Study the drawing (mm; zero at the part's minimum x, y, z) and answer. Coordinates: 2 decimals unless noted, no trailing zeros. Order: outer loops, then holes, each group sorted by start corner. A loop starts at its lowest first (then second) coordinate and runs counter-clockwise, first axis right, second up.
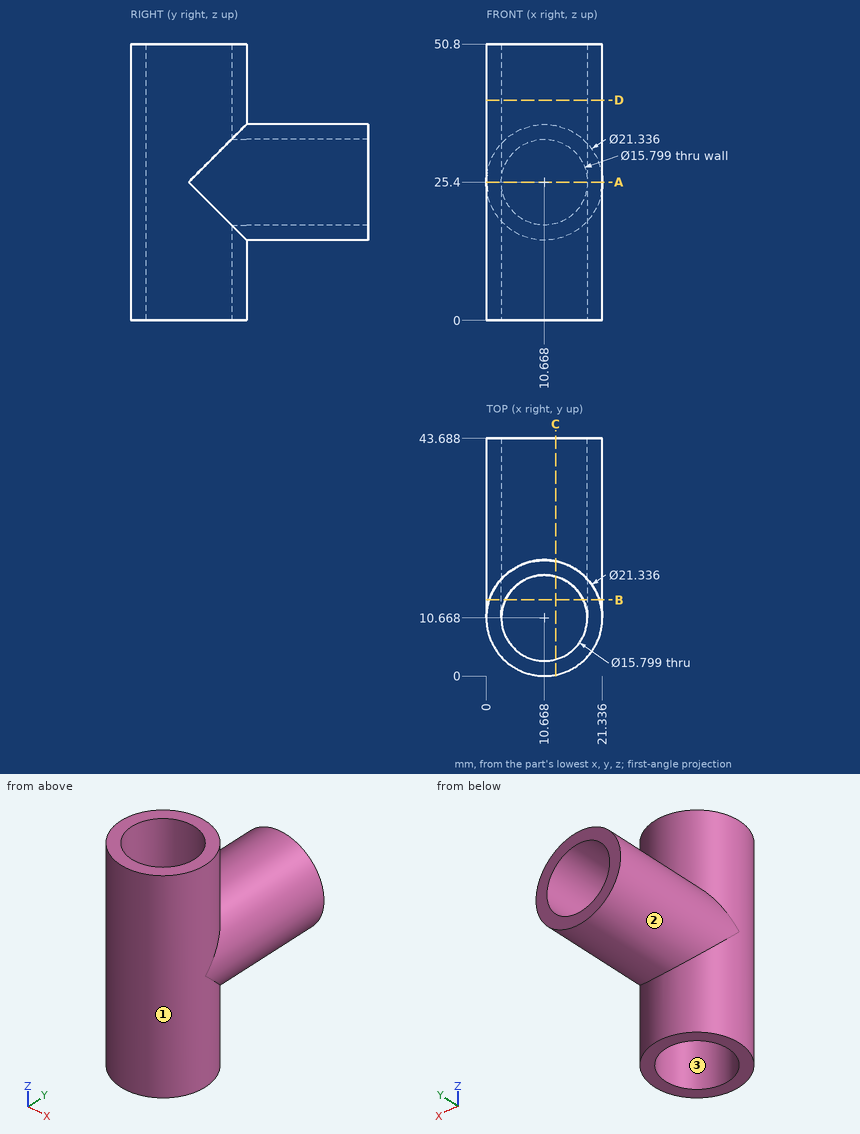
1) A cutting plane is placed at B-B, the plane y = 14. Determine the outline of the cut face in (x, z), and give its area (3 significant figures).
A:
outline: (0.53, 0) - (3.51, 0) - (3.51, 22.07) arc R7.9 cw to (3.51, 28.73) - (3.51, 50.8) - (0.53, 50.8) - (0.53, 28.73) arc R10.67 ccw to (0.53, 22.07) - close; (17.83, 0) - (20.8, 0) - (20.8, 22.07) arc R10.67 ccw to (20.8, 28.73) - (20.8, 50.8) - (17.83, 50.8) - (17.83, 28.73) arc R7.9 cw to (17.83, 22.07) - close
area: 300 mm2
2) A cutting plane is placed at D-D, the plane z = 40.5. Determine the outline of the cut face in (x, y).
A:
outline: circle Ø21.34 at (10.67, 10.67); hole circle Ø15.8 at (10.67, 10.67)
3) A cutting plane is placed at A-A, the plane z = 25.4. Determine the outline of the cut face in (x, y).
A:
outline: (0, 10.67) arc R10.67 ccw to (21.34, 10.67) - (21.34, 43.69) - (18.57, 43.69) - (18.57, 10.67) arc R7.9 cw to (2.77, 10.67) - (2.77, 43.69) - (0, 43.69) - close
4) Straight lines are drawn through the part: line 1 (Y direction, x = 11, z = 44) (1 decimal); line 2 (X direction, y = 24, z = 25.4); line 3 (X direction, y = 5, z = 9) (1 decimal). For each, find the intervals that lie inside material, in ascending order.
A:
line 1: y = 0 to 2.8, 18.6 to 21.3
line 2: x = 0 to 2.77, 18.57 to 21.34
line 3: x = 1.6 to 5.2, 16.2 to 19.7
5) A cutting plane is placed at C-C, the plane x = 12.75. Determine the outline of the cut face in (y, z) (1 decimal).
A:
outline: (0.2, 0) - (3, 0) - (3, 50.8) - (0.2, 50.8) - close; (18.3, 0) - (21.1, 0) - (21.1, 14.9) - (43.7, 14.9) - (43.7, 17.8) - (18.3, 17.8) - close; (18.3, 33) - (43.7, 33) - (43.7, 35.9) - (21.1, 35.9) - (21.1, 50.8) - (18.3, 50.8) - close
6) Determine the mould class of the marked faces 1, 2 and 3 for opening direction Y: pulls with the +Y half, pulls with the -Y half, needs draft (parallel to the pull), parting line crosses it, or undercut.
A:
face 1: parting line crosses it
face 2: needs draft
face 3: undercut
7) Flat-ended cylindrical pins translate along their axes: pin 1 Ø10 at (x, y) = (2.5, 25.5) entering from -Z; pin 2 Ø10 at (y, z) = (34, 39) entering from +X; pin 3 Ø5 at (x, y) = (18, 34.5) entering from -Z; pin 4 Ø12.5 at (x, y) = (10.668, 10.668) entering from -Z. Find the tip coordinate at first contact, or state that the pin passes through.
A:
pin 1: stops at z = 15.21
pin 2: stops at x = 16.98
pin 3: stops at z = 15.89
pin 4: passes through
